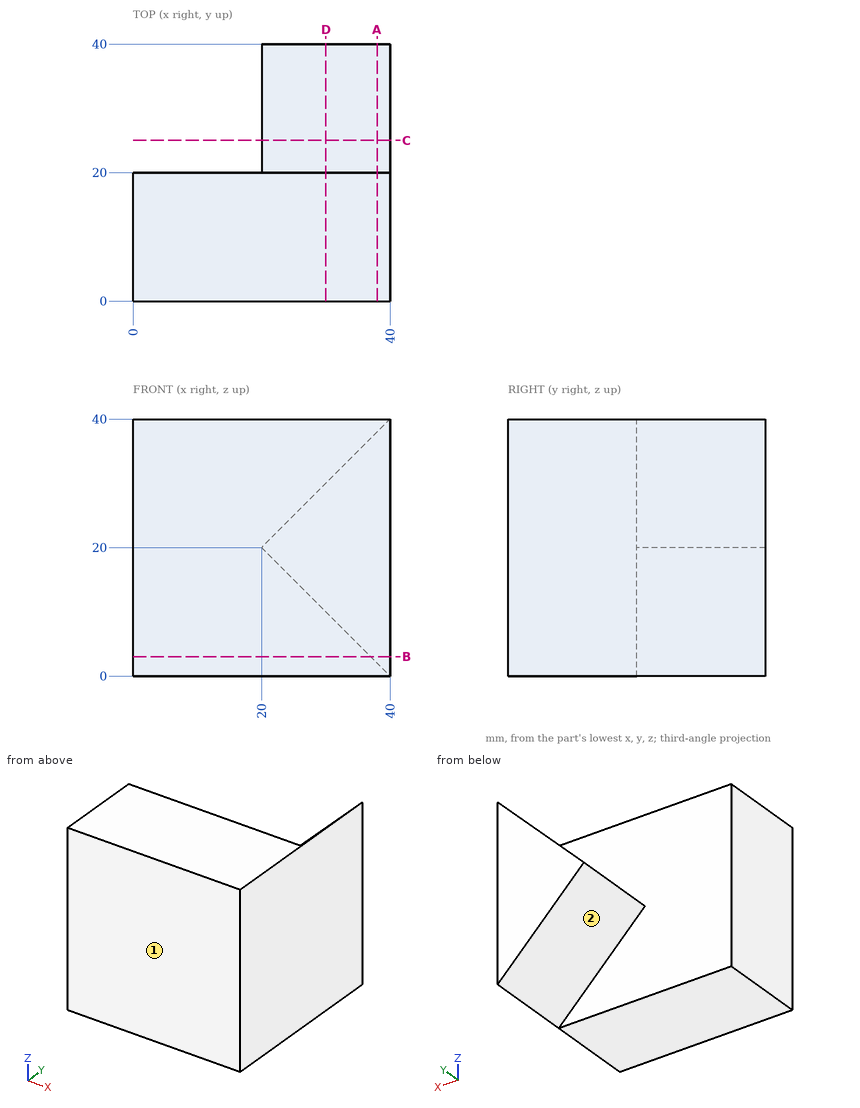
Source: three-view drawing plus pictorial views. Frame: mm from the lowest corner of the part. A direction names the side the tool comes from. Give positions to 0.01 mm unless a question says otherwise; leave off trailing zeros. Order: outer loops, then holes, each group sorted by start corner. A loop starts at its lowest first (then second) coordinate and runs counter-clockwise, first axis right, second up.
1. Section D-D on x = 30. Return the cut outline in (y, z).
Derived:
outline: (0, 0) - (20, 0) - (20, 10) - (40, 10) - (40, 30) - (20, 30) - (20, 40) - (0, 40) - close
2. Reachability of the marked faces 1 and 2 from +Z, -Z, +X, -X, +Y, -Y: full face, straight path, thin tool, end or side. Return the list, or none.
Derived:
face 1: +Z, -Z, +X, -X, -Y
face 2: -Z, -X, +Y
3. Section B-B on z = 3. Return the cut outline in (x, y).
Derived:
outline: (0, 0) - (40, 0) - (40, 40) - (37, 40) - (37, 20) - (0, 20) - close
4. Material intervals for L1, parallel to Y at x = 22.5, z = 4; L2, parallel to X at y = 24.5, z = 8.5; L3, parallel to Z at x = 33.5, y = 34, sorted ascending.
Derived:
L1: y = 0 to 20
L2: x = 31.5 to 40
L3: z = 6.5 to 33.5
5. Section A-A on x = 38. Return the cut outline in (y, z).
Derived:
outline: (0, 0) - (20, 0) - (20, 2) - (40, 2) - (40, 38) - (20, 38) - (20, 40) - (0, 40) - close
6. Section C-C on y = 25. Return the cut outline in (x, z).
Derived:
outline: (20, 20) - (40, 0) - (40, 40) - close
